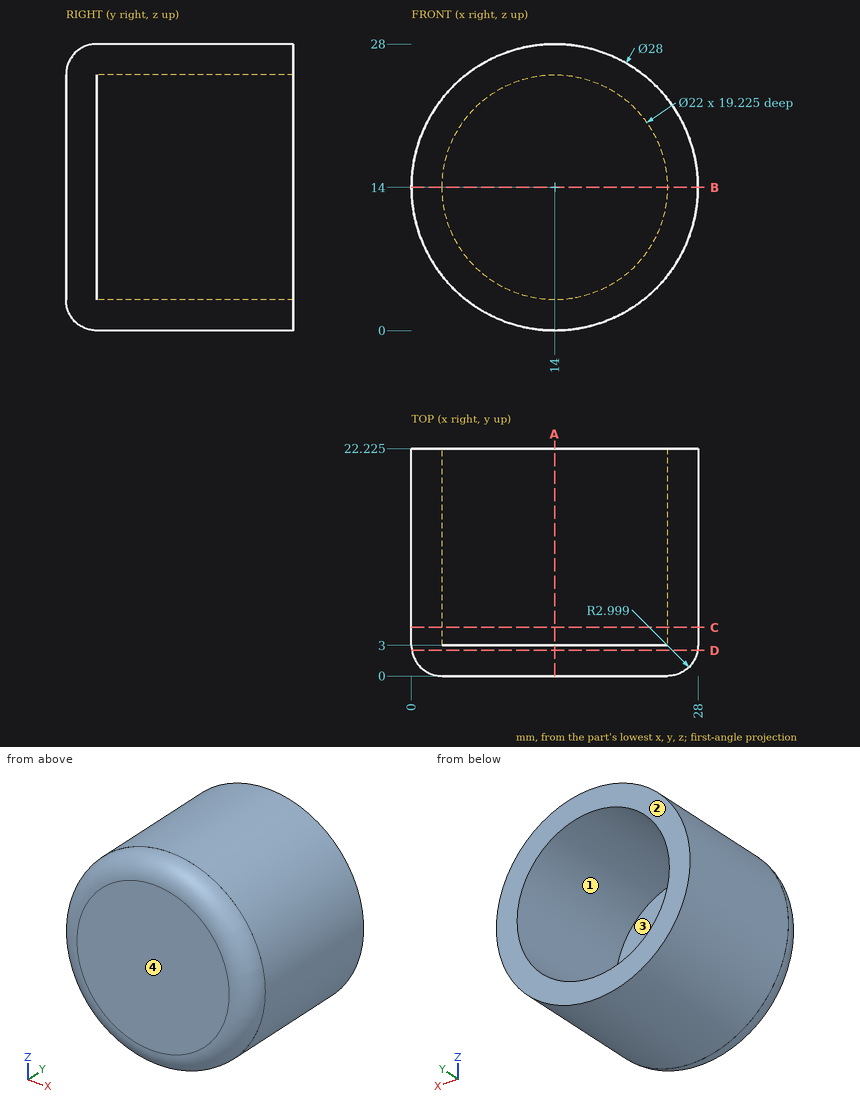
Input: dimensioned drawing with shaded views. Units: mm. Origin: part minimum x, y, z. A direction names the side the tool comes from. Coordinates: 2 decimals unless noted, no trailing zeros. Order: outer loops, then holes, each group sorted by start corner. A loop starts at its lowest first (then second) coordinate and runs counter-clockwise, first axis right, second up. Notation, with made-up numbers: (44.5, 76) - (87.5, 76) arc R21 ccw to (87.5, 85) - close; hole circle Ø8 at (62, 4.25). An arc over 180 degrees is marked (long way). Return JSON: item names as keys, results as strings. Group by question number.
1. Set-up query: the marked faces 3 and 4. Return all of +Z, -Z, +X, -X, +Y, -Y with unobstructed straight access to the full face (end or side cutting, diameter ignored); none if empty.
2. Cut plane A-A (x = 14). Output: boundary loops of the cut face in (y, z) (1 decimal).
3. Cut plane C-C (y = 4.75). Output: boundary loops of the cut face in (x, z).
4. Material intervals for line 1 along Z through (x, y) = (14, 13.5); line 2 along Y through (x, z) = (14, 17.25), sorted ascending. Write a range as [from, to].
5. Cut plane B-B (z = 14). Output: boundary loops of the cut face in (x, y) (1 decimal).
6. Pull-direction query (X, two-part tool) for the marked faces 1 and 2; classes: pulls with the +X half, pulls with the -X half, needs draft (parallel to the pull), parting line crosses it, or undercut.
7. Cut plane D-D (y = 2.5). Output: boundary loops of the cut face in (x, z), plus the area to 3 significant figures.
8. Pin query (flat end, axial travel): pin 1 (3 mm diameter, centred on x = 5, y = 9.5, fed in from +Z); pin 2 (10 mm diameter, centred on y = 10.5, z = 22.5, fed in from +X) (1 decimal); pin 3 (4 mm diameter, centred on x = 10, z = 22, fed in from +Y). Return the tip coordinate at first contact, or that it passes through.
Resolved:
{
 "1": {"face 3": "+Y", "face 4": "+Z, -Z, +X, -X, -Y"},
 "2": {"outline": "(0, 3) arc R3 ccw to (3, 0) - (22.2, 0) - (22.2, 3) - (3, 3) - (3, 25) - (22.2, 25) - (22.2, 28) - (3, 28) arc R3 ccw to (0, 25) - close"},
 "3": {"outline": "circle Ø28 at (14, 14); hole circle Ø22 at (14, 14)"},
 "4": {"line 1": "z = [0, 3], [25, 28]", "line 2": "y = [0, 3]"},
 "5": {"outline": "(0, 3) arc R3 ccw to (3, 0) - (25, 0) arc R3 ccw to (28, 3) - (28, 22.2) - (25, 22.2) - (25, 3) - (3, 3) - (3, 22.2) - (0, 22.2) - close"},
 "6": {"face 1": "undercut", "face 2": "needs draft"},
 "7": {"outline": "circle Ø27.92 at (14, 14)", "area": "612 mm²"},
 "8": {"pin 1": "stops at z = 25.82", "pin 2": "stops at x = 27.6", "pin 3": "stops at y = 3"}
}
